Source: CAD feature listing. Evaluate the final solid. Frame: model axes, mm. A direction names the side the tool comes from. Round coordinates to 2 decimals unless told otherwise and drop trailing zeros. Loops run counter-clockwise (first coordinate to the right, second up) from the corner with the lowest first, then second, coordinate; pieces in that order, holes last.
Item 1: Section query B-B on x = 100. Return loops of the section in (y, z), then the cut area to 3 significant figures.
Item 2: Ray query, L1, parallel to X at y = 3.5, z = 30.5; L2, parallel to Z at x = -112, y = 2.95; L3, parallel to Z at x = -64, y = 2.4. Return the intervals inside material, ascending.
Item 3: Access query for faces 1 (the cylindrical face through (122.281, 2.465, -11.906)), 2 (the cylindrical face through (77.25, 2.46, 14.76)). Directions: +Z, -Z, +X, -X, +Y, -Y. A direction counts if a zero-diameter tool reaches every point of the face in a straight line with its end or side. Return the directions, or none.
Item 4: Section query D-D on y = 3.3. Give the number of separate pieces and of enclosed holes in the cut face, then the cut area to 3 significant figures.
Item 5: Pull-direction query (Z, two-part tool) for faces 3 (the cylindrical face through (-143.997, 2.465, 14.236)), 4 (the flat face through (38, 5, -19)), 5 (the cylindrical face through (-122.406, 2.465, -11.781)), 6 (the cylindrical face through (-77.25, 2.46, 14.76)); classes: released by +Z, released by -Z, zero draft, split by the parting line, or undercut.
Item 6: Section query C-C on x = 31. Return loops of the section in (y, z), then the cut area to 3 significant figures.
Item 7: First-contact query: P1, Ø1, axis at y = 1, z = -61, coming from the -X side; P2, Ø1.5, axis at x = -70.5, y = 4, coming from the -Z side; P3, Ø2.5, axis at x = 144.5, y = 2.5, coming from the -Z side; P4, Ø4, axis at x = -112, z = -17.5, coming from the +Y side. Flat tips, straight axial feed; report the tip coordinate or a pass-through.
Item 8: Section query A-A on z = 14.5. Return loops of the section in (x, y), then the cut area to 3 significant figures.
```python
from build123d import *

# Parameters (mm, degrees)
SKETCH1_R               = 2.1
BOSS_EXTRUDE2_DEPTH     = 5
SKETCH2_W               = 324
SKETCH2_H               = 4
CUT_EXTRUDE1_DEPTH      = 1
CUT_EXTRUDE1_DEPTH_BACK = 6


with BuildPart() as part:
    # Sketch1 → Boss-Extrude2 (new body)
    with BuildSketch(Plane(origin=(0, 0, 0), x_dir=(1, 0, 0), z_dir=(0, 1, 0))):
        with BuildLine():
            Line((-112, 57.5), (-5, 57.5))
            ThreePointArc((-5, 57.5), (-1.464466094, 58.964466094), (0, 62.5))
            Line((0, 62.5), (0, 124.5))
            ThreePointArc((0, 124.5), (1.464466094, 128.035533906), (5, 129.5))
            Line((5, 129.5), (115, 129.5))
            ThreePointArc((115, 129.5), (118.535533906, 128.035533906), (120, 124.5))
            Line((120, 124.5), (120, 49.5))
            Line((120, 49.5), (120, 17.5))
            ThreePointArc((120, 17.5), (122.343145751, 11.843145751), (128, 9.5))
            Line((128, 9.5), (154, 9.5))
            ThreePointArc((154, 9.5), (159.656854249, 7.156854249), (162, 1.5))
            Line((162, 1.5), (162, -57.5))
            Line((162, -57.5), (-162, -57.5))
            Line((-162, -57.5), (-162, 1.5))
            ThreePointArc((-162, 1.5), (-159.656854249, 7.156854249), (-154, 9.5))
            Line((-154, 9.5), (-128, 9.5))
            ThreePointArc((-128, 9.5), (-122.343145751, 11.843145751), (-120, 17.5))
            Line((-120, 17.5), (-120, 49.5))
            ThreePointArc((-120, 49.5), (-117.656854249, 55.156854249), (-112, 57.5))
        make_face()
        with Locations((112, 49.5)):
            Circle(SKETCH1_R, mode=Mode.SUBTRACT)
        with Locations((112, 17.5)):
            Circle(SKETCH1_R, mode=Mode.SUBTRACT)
        with Locations((64, -30.5)):
            Circle(SKETCH1_R, mode=Mode.SUBTRACT)
        with Locations((64, 1.5)):
            Circle(SKETCH1_R, mode=Mode.SUBTRACT)
        with Locations((-112, 17.5)):
            Circle(SKETCH1_R, mode=Mode.SUBTRACT)
        with Locations((-112, 49.5)):
            Circle(SKETCH1_R, mode=Mode.SUBTRACT)
        with Locations((-64, 1.5)):
            Circle(SKETCH1_R, mode=Mode.SUBTRACT)
        with Locations((-64, -30.5)):
            Circle(SKETCH1_R, mode=Mode.SUBTRACT)
        with BuildLine():
            Line((8, 20.5), (8, -36.5))
            ThreePointArc((8, -36.5), (6.535533906, -40.035533906), (3, -41.5))
            Line((3, -41.5), (-3, -41.5))
            ThreePointArc((-3, -41.5), (-6.535533906, -40.035533906), (-8, -36.5))
            Line((-8, -36.5), (-8, 20.5))
            ThreePointArc((-8, 20.5), (-9.464466094, 24.035533906), (-13, 25.5))
            Line((-13, 25.5), (-37, 25.5))
            ThreePointArc((-37, 25.5), (-40.535533906, 26.964466094), (-42, 30.5))
            Line((-42, 30.5), (-42, 36.5))
            ThreePointArc((-42, 36.5), (-40.535533906, 40.035533906), (-37, 41.5))
            Line((-37, 41.5), (37, 41.5))
            ThreePointArc((37, 41.5), (40.535533906, 40.035533906), (42, 36.5))
            Line((42, 36.5), (42, 30.5))
            ThreePointArc((42, 30.5), (40.535533906, 26.964466094), (37, 25.5))
            Line((37, 25.5), (13, 25.5))
            ThreePointArc((13, 25.5), (9.464466094, 24.035533906), (8, 20.5))
        make_face(mode=Mode.SUBTRACT)
        with BuildLine():
            Line((132, -26.5), (89.247795496, -26.5))
            ThreePointArc((89.247795496, -26.5), (77.247795496, -14.5), (89.247795496, -2.5))
            Line((89.247795496, -2.5), (132, -2.5))
            ThreePointArc((132, -2.5), (144, -14.5), (132, -26.5))
        make_face(mode=Mode.SUBTRACT)
        with BuildLine():
            Line((-132, -26.5), (-89.247795496, -26.5))
            ThreePointArc((-89.247795496, -26.5), (-77.247795496, -14.5), (-89.247795496, -2.5))
            Line((-89.247795496, -2.5), (-132, -2.5))
            ThreePointArc((-132, -2.5), (-144, -14.5), (-132, -26.5))
        make_face(mode=Mode.SUBTRACT)
    extrude(amount=BOSS_EXTRUDE2_DEPTH)

    # Sketch2 → Cut-Extrude1 (cut, two sides)
    with BuildSketch(Plane(origin=(0, 5, 0), x_dir=(1, 0, 0), z_dir=(0, 1, 0))) as cut_extrude1_sk:
        with Locations((0, -55.5)):
            Rectangle(SKETCH2_W, SKETCH2_H)
    extrude(amount=CUT_EXTRUDE1_DEPTH, mode=Mode.SUBTRACT)
    extrude(cut_extrude1_sk.sketch, amount=-CUT_EXTRUDE1_DEPTH_BACK, mode=Mode.SUBTRACT)


solid = part.part
```
Data:
1. outline: (0, -129.5) - (5, -129.5) - (5, 2.5) - (0, 2.5) - close; (0, 26.5) - (5, 26.5) - (5, 53.5) - (0, 53.5) - close
1. area: 795 mm2
2. L1: x = -162 to -66.1, -61.9 to -8, 8 to 61.9, 66.1 to 162
2. L2: z = -57.5 to -51.6, -47.4 to -19.6, -15.4 to 2.5, 26.5 to 53.5
2. L3: z = -57.5 to -3.6, 0.6 to 28.4, 32.6 to 53.5
3. face 1: -Z, +X, +Y, -Y
3. face 2: +Y, -Y
4. separate pieces: 1
4. enclosed holes: 11
4. area: 35,100 mm2
5. face 3: undercut
5. face 4: zero draft
5. face 5: released by -Z
5. face 6: undercut
6. outline: (0, -129.5) - (5, -129.5) - (5, -41.5) - (0, -41.5) - close; (0, -25.5) - (5, -25.5) - (5, 53.5) - (0, 53.5) - close
6. area: 835 mm2
7. P1: stops at x = -0.42
7. P2: stops at z = -57.5
7. P3: stops at z = -9.5
7. P4: passes through
8. outline: (-162, 0) - (-144, 0) - (-144, 5) - (-162, 5) - close; (-77.25, 0) - (-8, 0) - (-8, 5) - (-77.25, 5) - close; (8, 0) - (77.25, 0) - (77.25, 5) - (8, 5) - close; (144, 0) - (162, 0) - (162, 5) - (144, 5) - close
8. area: 872 mm2
